Check sheet for the modelled part. Datum: model origin and axes. Units: mm. Face numbers are marked on the shaded views. Coordinates: 2 decimals unless noted, no trailing zeros. Loops run counter-clockwise (first coordinate to the right, second up) from the corner with the lowest first, then second, coordinate; pieces in that order, holes last. Notation, with made-up numbers: (28, 13.5) -> (55, 13.5) arc R28 ccw to (55, 44.5) -> close; hole circle Ø2 at (5.5, -7.75). An arc over 180 degrees is marked (long way). Use CSV: the item, a comma, the result in double quotes.
```python
from build123d import *

# Parameters (mm, degrees)
CROQUIS1_R              = 1.7
CROQUIS1_R_2            = 3.5
SALIENTE_EXTRUIR1_DEPTH = 40
REDONDEO1_R             = 6
CORTAR_EXTRUIR1_DEPTH   = 10
REDONDEO2_R             = 2


with BuildPart() as part:
    # Croquis1 → Saliente-Extruir1 (new body, symmetric)
    with BuildSketch(Plane.XY):
        with BuildLine():
            Line((-78.419273977, 20.002017027), (-87.494309747, 2.17945476))
            ThreePointArc((-87.494309747, 2.17945476), (-92.663415431, -3.564512453), (-91.0588222, 3.994461914))
            Line((-91.0588222, 3.994461914), (-81.98378643, 21.817024181))
            ThreePointArc((-81.98378643, 21.817024181), (3.624504321, 72.000435004), (85.015988263, 15.232657976))
            Line((85.015988263, 15.232657976), (88.837814169, 5.991789686))
            ThreePointArc((88.837814169, 5.991789686), (91.444687267, -5.544520974), (85.141466854, 4.463059324))
            Line((85.141466854, 4.463059324), (81.319640948, 13.703927614))
            ThreePointArc((81.319640948, 13.703927614), (3.466917176, 68.003540423), (-78.419273977, 20.002017027))
        make_face()
        with Locations((-90.848408277, 0)):
            Circle(CROQUIS1_R, mode=Mode.SUBTRACT)
        with Locations((89.151591723, 0)):
            Circle(CROQUIS1_R_2, mode=Mode.SUBTRACT)
    extrude(amount=SALIENTE_EXTRUIR1_DEPTH, both=True)

    # Redondeo1
    redondeo1_edges = [part.edges().sort_by_distance(p)[0] for p in [
        (-87.494309747, 2.17945476, 0),
        (-91.0588222, 3.994461914, 0),
        (88.837814169, 5.991789686, 0),
        (85.141466854, 4.463059324, 0),
    ]]
    fillet(redondeo1_edges, radius=REDONDEO1_R)

    # Croquis2 → Cortar-Extruir1 (cut)
    with BuildSketch(Plane(origin=(0, 0, -40), x_dir=(-1, 0, 0), z_dir=(0, 0, -1))):
        with BuildLine():
            Line((89.908153773, 6.254272257), (86.343641319, 4.439265103))
            ThreePointArc((86.343641319, 4.439265103), (86.930196271, 2.608758116), (86.907794022, 0.686701749))
            ThreePointArc((86.907794022, 0.686701749), (92.663415431, -3.564512453), (92.611013947, 3.590713195))
            ThreePointArc((92.611013947, 3.590713195), (91.043465794, 4.703185814), (89.908153773, 6.254272257))
        make_face()
        with BuildLine():
            Line((-87.581420372, 9.029649048), (-83.885073056, 7.500918685))
            ThreePointArc((-83.885073056, 7.500918685), (-84.338136431, 5.037582192), (-83.746071903, 2.603911571))
            ThreePointArc((-83.746071903, 2.603911571), (-91.444687267, -5.544520974), (-91.138766534, 5.661372296))
            ThreePointArc((-91.138766534, 5.661372296), (-89.000661668, 6.965903123), (-87.581420372, 9.029649048))
        make_face()
    cortar_extruir1 = extrude(amount=-CORTAR_EXTRUIR1_DEPTH, mode=Mode.SUBTRACT)

    # Simetría1: Cortar-Extruir1 across plane
    add(cortar_extruir1.mirror(Plane.XY), mode=Mode.SUBTRACT)

    # Redondeo2
    redondeo2_edges = [part.edges().sort_by_distance(p)[0] for p in [
        (85.651591723, 0, 30),
        (85.651591723, 0, -30),
    ]]
    fillet(redondeo2_edges, radius=REDONDEO2_R)


solid = part.part
```
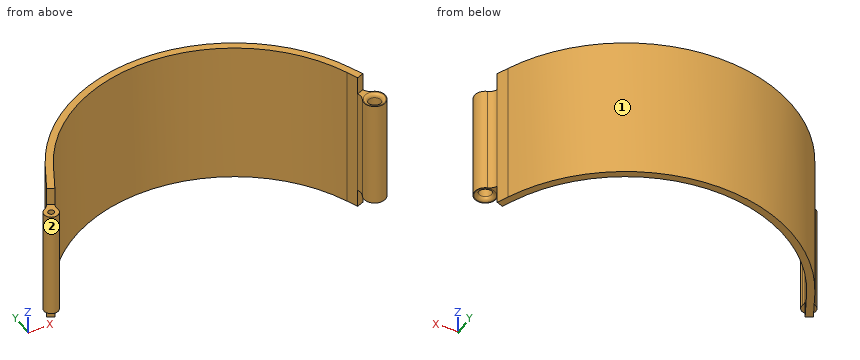
1) Cross-section at D-D on x = -46. Record the boundary of the cut face in (y, z).
Answer below:
outline,"(55.09, -40) -> (59.75, -40) -> (59.75, 40) -> (55.09, 40) -> close"
2) Draft check along X on the marked faces 1 and 2. Enter one of: released by +X, released by -X, zero draft, split by the parting line, or undercut.
Answer below:
face 1,"split by the parting line"
face 2,"undercut"
3) Go/stop test with flat-tipped pins: pin 1 Ø10 at (x, z) = (-38.5, 25.5) entering from -Y; pin 2 Ø1.5 at (x, z) = (4, -24) entering from +Y; pin 3 Ø4.5 at (x, y) = (-90.85, 0) entering from +Z. Record where each tip stops, or that it passes through.
Answer below:
pin 1,"stops at y = 56.57"
pin 2,"stops at y = 72.01"
pin 3,"stops at z = 30"
4) Thickness scan on line 1 along X through (y, z) = (0, -15.5); line 2 along X through (y, z) = (47, 16); line 3 along X through (y, z) = (4, -9). Record the ranges inside material, lowest first. Write a range as from..to.
Answer below:
line 1,"x = -94.85..-92.55, -89.15..-86.85, 83.15..85.65, 92.65..95.15"
line 2,"x = -63.12..-57.14, 57.14..63.12"
line 3,"x = -91.9..-86.55, 84.22..93.62"
5) Cross-section at C-C on x = 40.5. Record the boundary of the cut face in (y, z).
Answer below:
outline,"(58.2, -40) -> (62.68, -40) -> (62.68, 40) -> (58.2, 40) -> close"
6) Cross-section at A-A on y = 39. Record the boundary of the cut face in (x, z), and give its area (3 significant figures).
Answer below:
outline,"(-70.65, -40) -> (-65.36, -40) -> (-65.36, 40) -> (-70.65, 40) -> close; (65.36, -40) -> (70.65, -40) -> (70.65, 40) -> (65.36, 40) -> close"
area,"847 mm²"
7) Cross-section at B-B on z = 4. Record the boundary of the cut face in (x, y), and give its area (3 significant figures).
Answer below:
outline,"(-92.61, 3.59) arc R4 ccw (long way) to (-86.91, 0.69) arc R6 cw to (-86.34, 4.44) -> (-78.42, 20) arc R88 cw to (81.32, 13.7) -> (83.89, 7.5) arc R6 cw to (83.75, 2.6) arc R6 ccw (long way) to (91.14, 5.66) arc R6 cw to (87.58, 9.03) -> (85.02, 15.23) arc R92 ccw to (-81.98, 21.82) -> (-89.91, 6.25) arc R6 cw to start; hole circle Ø3.4 at (-90.85, 0); hole circle Ø7 at (89.15, 0)"
area,"1,060 mm²"
